Check sheet for the modelled part. Datum: model origin and axes. Units: mm. A direction names the side the tool comes from. Round coordinates to 2 decimals unless told otherwise and drop trailing zeros. Write each loop counter-clockwise with the first axis right and the second up, starting at its lowest first coordinate (ties: lowest second). Pieces come first, ordered by that corner, then holes. Notation, with made-up numbers: M -17.75,-37 L 24.25,-37 A10 cw 24.25,-18 Z; hole C -39,68.25 d2. An arc over 180 degrees is marked long. Answer in a Markdown table with one row per item.
```python
from build123d import *

# Parameters (mm, degrees)
SKETCH1_W           = 43
SKETCH1_H           = 2
BOSS_EXTRUDE1_DEPTH = 43
SKETCH1_3_W         = 43
SKETCH1_3_H         = 74
BOSS_EXTRUDE2_DEPTH = 29.5
CUT_EXTRUDE1_REACH  = 78.885
SKETCH2_R           = 12.5
SKETCH2_R_2         = 1.75
CUT_EXTRUDE2_REACH  = 62.665
SKETCH1_4_R         = 2.75
LPATTERN1_COUNT     = 2
LPATTERN1_PITCH     = 11.5
LPATTERN1_COL_COUNT = 2
LPATTERN1_COL_PITCH = 11.5
SKETCH3_W           = 43
SKETCH3_H           = 12
CUT_EXTRUDE3_DEPTH  = 27.5


with BuildPart() as part:
    # Sketch1 → Boss-Extrude1 (new body)
    with BuildSketch(Plane(origin=(0, 0, 0), x_dir=(1, 0, 0), z_dir=(0, 1, 0))):
        with Locations((0, 24)):
            Rectangle(SKETCH1_W, SKETCH1_H)
    extrude(amount=BOSS_EXTRUDE1_DEPTH)

    # Sketch1_3 → Boss-Extrude2 (add)
    with BuildSketch(Plane(origin=(0, 0, 0), x_dir=(1, 0, 0), z_dir=(0, 1, 0))):
        Rectangle(SKETCH1_3_W, SKETCH1_3_H)
    extrude(amount=-BOSS_EXTRUDE2_DEPTH)

    # Sketch2 → Cut-Extrude1 (cut, up to next)
    with BuildSketch(Plane.XY.offset(-23), mode=Mode.PRIVATE) as cut_extrude1_sk1:
        with Locations((0, 21.5)):
            Circle(SKETCH2_R)
    cut_extrude1_tool1 = extrude(cut_extrude1_sk1.sketch, amount=-CUT_EXTRUDE1_REACH, mode=Mode.PRIVATE) & part.part
    # Sketch2 → Cut-Extrude1 (cut, up to next)
    with BuildSketch(Plane.XY.offset(-23), mode=Mode.PRIVATE) as cut_extrude1_sk2:
        with Locations((-15.5, 37)):
            Circle(SKETCH2_R_2)
    cut_extrude1_tool2 = extrude(cut_extrude1_sk2.sketch, amount=-CUT_EXTRUDE1_REACH, mode=Mode.PRIVATE) & part.part
    # Sketch2 → Cut-Extrude1 (cut, up to next)
    with BuildSketch(Plane.XY.offset(-23), mode=Mode.PRIVATE) as cut_extrude1_sk3:
        with Locations((15.5, 37)):
            Circle(SKETCH2_R_2)
    cut_extrude1_tool3 = extrude(cut_extrude1_sk3.sketch, amount=-CUT_EXTRUDE1_REACH, mode=Mode.PRIVATE) & part.part
    # Sketch2 → Cut-Extrude1 (cut, up to next)
    with BuildSketch(Plane.XY.offset(-23), mode=Mode.PRIVATE) as cut_extrude1_sk4:
        with Locations((15.5, 6)):
            Circle(SKETCH2_R_2)
    cut_extrude1_tool4 = extrude(cut_extrude1_sk4.sketch, amount=-CUT_EXTRUDE1_REACH, mode=Mode.PRIVATE) & part.part
    # Sketch2 → Cut-Extrude1 (cut, up to next)
    with BuildSketch(Plane.XY.offset(-23), mode=Mode.PRIVATE) as cut_extrude1_sk5:
        with Locations((-15.5, 6)):
            Circle(SKETCH2_R_2)
    cut_extrude1_tool5 = extrude(cut_extrude1_sk5.sketch, amount=-CUT_EXTRUDE1_REACH, mode=Mode.PRIVATE) & part.part
    add(cut_extrude1_tool1.solids().sort_by_distance((0, 21.5, -23))[0], mode=Mode.SUBTRACT)
    add(cut_extrude1_tool2.solids().sort_by_distance((-15.5, 37, -23))[0], mode=Mode.SUBTRACT)
    add(cut_extrude1_tool3.solids().sort_by_distance((15.5, 37, -23))[0], mode=Mode.SUBTRACT)
    add(cut_extrude1_tool4.solids().sort_by_distance((15.5, 6, -23))[0], mode=Mode.SUBTRACT)
    add(cut_extrude1_tool5.solids().sort_by_distance((-15.5, 6, -23))[0], mode=Mode.SUBTRACT)

    # Sketch1_4 → Cut-Extrude2 (cut, up to next)
    with BuildSketch(Plane(origin=(0, 0, 0), x_dir=(1, 0, 0), z_dir=(0, 1, 0)), mode=Mode.PRIVATE) as cut_extrude2_sk1:
        with Locations(Location((0, 31, 0), (0, 0, 270))):
            Circle(SKETCH1_4_R)
    cut_extrude2_tool1 = extrude(cut_extrude2_sk1.sketch, amount=-CUT_EXTRUDE2_REACH, mode=Mode.PRIVATE) & part.part
    # Sketch1_4 → Cut-Extrude2 (cut, up to next)
    with BuildSketch(Plane(origin=(0, 0, 0), x_dir=(1, 0, 0), z_dir=(0, 1, 0)), mode=Mode.PRIVATE) as cut_extrude2_sk2:
        with Locations(Location((0, -31, 0), (0, 0, 270))):
            Circle(SKETCH1_4_R)
    cut_extrude2_tool2 = extrude(cut_extrude2_sk2.sketch, amount=-CUT_EXTRUDE2_REACH, mode=Mode.PRIVATE) & part.part
    cut_extrude2_1 = cut_extrude2_tool1.solids().sort_by_distance((0, 0, -31))[0]
    add(cut_extrude2_1, mode=Mode.SUBTRACT)
    cut_extrude2_2 = cut_extrude2_tool2.solids().sort_by_distance((0, 0, 31))[0]
    add(cut_extrude2_2, mode=Mode.SUBTRACT)
    cut_extrude2 = cut_extrude2_1 + cut_extrude2_2  # Cut-Extrude2 as one shape, for the pattern or mirror that repeats it

    # LPattern1: Cut-Extrude2 ×2
    with Locations(*[(i * LPATTERN1_PITCH, 0, 0) for i in range(1, LPATTERN1_COUNT)]):
        add(cut_extrude2, mode=Mode.SUBTRACT)

    # LPattern1 col: Cut-Extrude2 ×2
    with Locations(*[(-i * LPATTERN1_COL_PITCH, 0, 0) for i in range(1, LPATTERN1_COL_COUNT)]):
        add(cut_extrude2, mode=Mode.SUBTRACT)

    # Sketch3 → Cut-Extrude3 (cut)
    with BuildSketch(Plane(origin=(0, 0, 0), x_dir=(1, 0, 0), z_dir=(0, 1, 0))):
        with Locations((0, -31)):
            Rectangle(SKETCH3_W, SKETCH3_H)
        with Locations((0, 31)):
            Rectangle(SKETCH3_W, SKETCH3_H)
    extrude(amount=-CUT_EXTRUDE3_DEPTH, mode=Mode.SUBTRACT)


solid = part.part
```
1. Access from +Z, -Z, +X, -X, +Y, -Y to the whole of each face (thin tool, end or side, straight path). Record for faces 1 (the face through (0, -27.5, -34)), 2 (the face through (0, -14, 25)), 3 (the face through (0.121, -28.486, 28.253)).
Found:
| item | result |
|---|---|
| face 1 | -Z, +X, -X, +Y |
| face 2 | +Z, +X, -X, +Y |
| face 3 | +Y, -Y |
2. Section check A-A, the plane x = 15.5. Record the cut outline in (y, z).
Found:
| item | result |
|---|---|
| outline | M -29.5,-37 L -27.5,-37 L -27.5,-25 L 4.25,-25 L 4.25,-23 L 0,-23 L 0,25 L -27.5,25 L -27.5,37 L -29.5,37 Z; M 7.75,-25 L 35.25,-25 L 35.25,-23 L 7.75,-23 Z; M 38.75,-25 L 43,-25 L 43,-23 L 38.75,-23 Z |
3. Section check C-C, the plane y = 21.5. Record the cut outline in (x, z), and give its area (3 significant figures).
Found:
| item | result |
|---|---|
| outline | M -21.5,-25 L -12.5,-25 L -12.5,-23 L -21.5,-23 Z; M 12.5,-25 L 21.5,-25 L 21.5,-23 L 12.5,-23 Z |
| area | 36.0 mm2 |
4. Draft check along X on faces 4 (the face through (21.5, -12, 0)), 5 (the face through (0, 0, 1)), 6 (the face through (16.31, 4.45, -23.99)), 7 (the face through (-21.5, -12, 0)). Enter one of: +X half, -X half, draft (parallel to the pull), parting line (faces both ways), or undercut.
Found:
| item | result |
|---|---|
| face 4 | +X half |
| face 5 | draft |
| face 6 | undercut |
| face 7 | -X half |
5. Section check D-D, the plane x = 0. Record the cut outline in (y, z).
Found:
| item | result |
|---|---|
| outline | M -29.5,-37 L -27.5,-37 L -27.5,-33.75 L -29.5,-33.75 Z; M -29.5,-28.25 L -27.5,-28.25 L -27.5,-25 L 9,-25 L 9,-23 L 0,-23 L 0,25 L -27.5,25 L -27.5,28.25 L -29.5,28.25 Z; M -29.5,33.75 L -27.5,33.75 L -27.5,37 L -29.5,37 Z; M 34,-25 L 43,-25 L 43,-23 L 34,-23 Z |
6. Go/stop test with flat-tipped pins: pin 1 (4 mm diameter, centred on x = 15.5, y = 37, fed in from -Z); pin 2 (9.5 mm diameter, centred on x = 5.5, z = -31.5, fed in from +Y); pin 3 (14 mm diameter, centred on x = -2.5, y = -18, fed in from +Z). Record where each tip stops, or that it passes through.
Found:
| item | result |
|---|---|
| pin 1 | stops at z = -25 |
| pin 2 | stops at y = -27.5 |
| pin 3 | stops at z = 25 |
7. Scan lines: L1, parallel to Y at x = 15.5, z = -24.2; L2, parallel to X at y = -27.95, z = 31; L3, parallel to Y at x = 12.5, z = 16.5. Record each from-to range of solid material in increasing order.
Found:
| item | result |
|---|---|
| L1 | y = -29.5 to 4.25, 7.75 to 35.25, 38.75 to 43 |
| L2 | x = -21.5 to -14.25, -8.75 to -2.75, 2.75 to 8.75, 14.25 to 21.5 |
| L3 | y = -29.5 to 0 |
8. Section check B-B, the plane z = -31. Record the cut outline in (x, y).
Found:
| item | result |
|---|---|
| outline | M -21.5,-29.5 L -14.25,-29.5 L -14.25,-27.5 L -21.5,-27.5 Z; M -8.75,-29.5 L -2.75,-29.5 L -2.75,-27.5 L -8.75,-27.5 Z; M 2.75,-29.5 L 8.75,-29.5 L 8.75,-27.5 L 2.75,-27.5 Z; M 14.25,-29.5 L 21.5,-29.5 L 21.5,-27.5 L 14.25,-27.5 Z |
